```python
from build123d import *

# Parameters (mm, degrees)
F0_R     = 3
F0_R_2   = 2
F1_DEPTH = 1.5


with BuildPart() as f1:
    # F0 (on Front) → F1 (new body)
    with BuildSketch(Plane.XZ):
        with BuildLine():
            ThreePointArc((3.5, 25), (0, 28.5), (-3.5, 25))
            Line((-3.5, 25), (-3.5, 8.587782))
            ThreePointArc((-3.5, 8.587782), (-3.898568, 5.792697), (-5.0625, 3.220418))
            ThreePointArc((-5.0625, 3.220418), (0, -6), (5.0625, 3.220418))
            ThreePointArc((5.0625, 3.220418), (3.898568, 5.792697), (3.5, 8.587782))
            Line((3.5, 8.587782), (3.5, 25))
        make_face()
        Circle(F0_R, mode=Mode.SUBTRACT)
        with Locations((0, 25)):
            Circle(F0_R_2, mode=Mode.SUBTRACT)
    extrude(amount=F1_DEPTH)


solid = f1.part
```
Check sheet for the modelled part. Datum: model origin and axes. Units: mm. Round coordinates to 2 decimals unless told otherwise and drop trailing zeros. Order: outer loops, then holes, each group sorted by start corner. A loop starts at its lowest first (then second) coordinate and runs counter-clockwise, first axis right, second up. Notation, with made-up numbers: (-4.5, 29) - (12.5, 29) arc R31 ccw to (12.5, 62) - close; hole circle Ø1 at (79.25, 75). An arc over 180 degrees is marked (long way). Answer as CSV lines item,"result". Start each with the question number.
1) Section check B-B (z = 0). Record the cut outline in (x, y), then the cut area to 3 significant figures.
2) Section check A-A (y = -0.45). Record the cut outline in (x, z), then the cut area to 3 significant figures.
3) Section check D-D (z = 14). Record the cut outline in (x, y).
4) Draft check along X on faces 1 (the face through (3.5, -1, 17)), 2 (the face through (-3, -1, 0)), 3 (the face through (-3.5, -1, 17)). Enter one of: +X half, -X half, draft (parallel to the pull), parting line (faces both ways), or undercut.
5) Scan lines: probe 1 along Z at (x, y) = (0, -1); probe 2 along Z at (x, y) = (0.5, -0.55); probe 3 along X at (y, z) = (-0.85, 17.5). Record each from-to range of solid material in increasing order.
6) Section check C-C (x = 0). Record the cut outline in (y, z), then the cut area to 4 significant figures.
7) Depth check by flat-ended pin: pin 1 (0.8 mm diameter, centred on y = -1, z = 19, fed in from -X); pin 2 (3.5 mm diameter, centred on x = 0, z = 0, fed in from -Y). Enter the tip coordinate at first touch or a pass-through.
Determined:
1,outline,"(-6, -1.5) - (-3, -1.5) - (-3, 0) - (-6, 0) - close; (3, -1.5) - (6, -1.5) - (6, 0) - (3, 0) - close"
1,area,"9.00 mm^2"
2,outline,"(-5.06, 3.22) arc R6 ccw (long way) to (5.06, 3.22) arc R10 cw to (3.5, 8.59) - (3.5, 25) arc R3.5 ccw to (-3.5, 25) - (-3.5, 8.59) arc R10 cw to start; hole circle Ø6 at (0, 0); hole circle Ø4 at (0, 25)"
2,area,"230 mm^2"
3,outline,"(-3.5, -1.5) - (3.5, -1.5) - (3.5, 0) - (-3.5, 0) - close"
4,face 1,"+X half"
4,face 2,"undercut"
4,face 3,"-X half"
5,probe 1,"-6 to -3, 3 to 23, 27 to 28.5"
5,probe 2,"-5.98 to -2.96, 2.96 to 23.06, 26.94 to 28.46"
5,probe 3,"-3.5 to 3.5"
6,outline,"(-1.5, -6) - (0, -6) - (0, -3) - (-1.5, -3) - close; (-1.5, 3) - (0, 3) - (0, 23) - (-1.5, 23) - close; (-1.5, 27) - (0, 27) - (0, 28.5) - (-1.5, 28.5) - close"
6,area,"36.75 mm^2"
7,pin 1,"x = -3.5"
7,pin 2,"through"
